CAD build for the part. Positions are in the model's coordinates, mm. A direction names the side the tool comes from. Coordinates: 2 decimals unless noted, no trailing zeros. Loops run counter-clockwise (first coordinate to the right, second up) from the corner with the lowest first, then second, coordinate; pieces in that order, holes last. Notation, with made-up numbers: (75.5, 80.25) -> (126.5, 80.25) arc R26 cw to (126.5, 108.25) -> close; hole circle Ø11 at (34, 21). An arc over 180 degrees is marked (long way). Write item = value, one per line. Start each with the question number.
(1) Flat gauge pins, fed straight in: P1, Ø16, axis at y = -4, z = 5.5, coming from the +X side; P2, Ø9.5, axis at y = -0.5, z = -7.5, coming from the -X side; P3, Ø6, axis at x = -18, z = -11.5, coming from the -Y side. Where does each tip first touch, or does it go through?
(2) Band-saw the part on A-A (x = -7). Write the cut outline in (y, z).
(3) Tool access for faces 1 (the face through (-30.5, 20, 7)), 2 (the face through (10, -11, 23)), 3 (the face through (-0.986, 7.91, -10.316)): list every direction of +Z, -Z, +X, -X, +Y, -Y with a clear straight run to the whole face (end or side of a thin tool).
(4) Pull direction Z, two halves, no side cores. Call faces 4 (the face through (-33.83, 18.163, -4.033)), 5 (the face through (-25, 23.43, 7.73)), 6 (the face through (-27, -10, -9)), 7 (the face through (-23.534, 13.384, -17.455)): +Z half, -Z half, draft (parallel to the pull), parting line (faces both ways), or undercut.
(5) Drill centre lines: line 1 (Y direction, x = -6.75, z = 0); line 2 (Z direction, x = -24, y = -9.5); line 3 (Y direction, x = -12, z = -7.5). Where is each one in solid material? Low to high. Write a range as from..to.
(6) Band-saw the part on B-B (x = 4). Write the cut outline in (y, z).
```python
from build123d import *


with BuildPart() as part:
    # Esquisse1 → R_volution1 (revolve)
    with BuildSketch(Plane.XY, mode=Mode.PRIVATE) as r_volution1_sk:
        Polygon((0, 10.5), (-18, 10.5), (-21, 13), (0, 13), align=None)
    revolve(r_volution1_sk.sketch.rotate(Axis((-90.5, 0, 0), (1, 0, 0)), 90), axis=Axis((-90.5, 0, 0), (1, 0, 0)))

    # Esquisse2 → R_volution4 (revolve)
    with BuildSketch(Plane.XY, mode=Mode.PRIVATE) as r_volution4_sk:
        with BuildLine():
            Line((-2, 13), (-2, 16))
            Line((-2, 16), (-22, 16))
            ThreePointArc((-22, 16), (-25.050730834, 18.263813026), (-23.768106875, 21.839660313))
            Line((-23.768106875, 21.839660313), (-20.027737076, 24.33324018))
            ThreePointArc((-20.027737076, 24.33324018), (-18.703156838, 24.95844884), (-17.254236095, 25.172988708))
            Line((-17.254236095, 25.172988708), (10, 25.172988708))
            Line((10, 25.172988708), (10, 28))
            Line((10, 28), (-22, 28))
            Line((-22, 28), (-22, 26.5))
            Line((-22, 26.5), (-25, 26.5))
            Line((-25, 26.5), (-25, 24.5))
            Line((-25, 24.5), (-27.5, 24.5))
            Line((-27.5, 24.5), (-27.5, 22.5))
            Line((-27.5, 22.5), (-30.5, 22.5))
            Line((-30.5, 22.5), (-30.5, 20.672988708))
            Line((-30.5, 20.672988708), (-34, 18.5))
            Line((-34, 18.5), (-34, 16))
            Line((-34, 16), (-29, 16))
            Line((-29, 16), (-29, 14.5))
            Line((-29, 14.5), (-27, 14.5))
            Line((-27, 14.5), (-27, 13))
            Line((-27, 13), (-2, 13))
        make_face()
    revolve(r_volution4_sk.sketch.rotate(Axis((-35.5, 0, 0), (1, 0, 0)), 90), axis=Axis((-35.5, 0, 0), (1, 0, 0)))


solid = part.part
```
Findings below:
q1.P1 = 0
q1.P2 = -20.12
q1.P3 = -26.68
q2.outline = circle Ø56 at (0, 0); circle Ø32 at (0, 0); hole circle Ø50.35 at (0, 0); hole circle Ø21 at (0, 0)
q3.face_1 = -X
q3.face_2 = +Z, -Z, +X, +Y, -Y
q3.face_3 = +X
q4.face_4 = parting line
q4.face_5 = draft
q4.face_6 = undercut
q4.face_7 = undercut
q5.line_1 = -28..-25.17, -16..-10.5, 10.5..16, 25.17..28
q5.line_2 = -24.74..-19.48, -13.74..-8.87, 8.87..13.74, 19.48..24.74
q5.line_3 = -26.98..-24.03, -14.13..-7.35, 7.35..14.13, 24.03..26.98
q6.outline = circle Ø56 at (0, 0); hole circle Ø50.35 at (0, 0)
